from build123d import *

# Parameters (mm, degrees)
SKETCH1_W           = 31.75
SKETCH1_H           = 12.7
SKETCH1_W_2         = 30
SKETCH1_H_2         = 7
BOSS_EXTRUDE1_DEPTH = 13
SKETCH4_R           = 1.778
CUT_EXTRUDE3_DEPTH  = 14
SKETCH5_W           = 21
SKETCH5_H           = 41
CUT_EXTRUDE4_DEPTH  = 10
SKETCH6_R           = 7.112
CUT_EXTRUDE5_DEPTH  = 4
SKETCH7_W           = 31.75
SKETCH7_H           = 12.7
CUT_EXTRUDE6_DEPTH  = 6.35
SKETCH8_R           = 1.778
CUT_EXTRUDE7_DEPTH  = 7.65
SKETCH10_R          = 1.905
CUT_EXTRUDE8_DEPTH  = 14
SKETCH11_R          = 3.302
CUT_EXTRUDE9_DEPTH  = 9.525
SKETCH13_W          = 9.525
SKETCH13_H          = 12.7
SKETCH13_R          = 1.778
BOSS_EXTRUDE2_DEPTH = 13
BOSS_EXTRUDE3_DEPTH = 13
SKETCH18_R          = 1.8415
CUT_EXTRUDE10_DEPTH = 14
FILLET1_R           = 9.525
FILLET2_R           = 3.175
FILLET3_R           = 3.175


with BuildPart() as part:
    # Sketch1 → Boss-Extrude1 (new body)
    with BuildSketch(Plane.XY):
        Polygon((31.75, 12.7), (31.75, 0), (31.75, -28.65), (61.75, -28.65), (61.75, 0), (61.75, 12.7), (61.75, 41.35), (31.75, 41.35), align=None)
        with Locations((15.875, 6.35)):
            Rectangle(SKETCH1_W, SKETCH1_H)
        with Locations((46.75, -32.15)):
            Rectangle(SKETCH1_W_2, SKETCH1_H_2)
    extrude(amount=BOSS_EXTRUDE1_DEPTH)

    # Sketch4 → Cut-Extrude3 (cut, through all)
    with BuildSketch(Plane.XY.offset(13)):
        with Locations((41.75, 22.199999832)):
            Circle(SKETCH4_R)
        with Locations((51.75, 22.199999832)):
            Circle(SKETCH4_R)
        with Locations((41.75, -27.800000168)):
            Circle(SKETCH4_R)
        with Locations((51.75, -27.800000168)):
            Circle(SKETCH4_R)
    extrude(amount=-CUT_EXTRUDE3_DEPTH, mode=Mode.SUBTRACT)

    # Sketch5 → Cut-Extrude4 (cut)
    with BuildSketch(Plane.XY.offset(13)):
        with Locations((46.75, -2.800000024)):
            Rectangle(SKETCH5_W, SKETCH5_H)
    extrude(amount=-CUT_EXTRUDE4_DEPTH, mode=Mode.SUBTRACT)

    # Sketch6 → Cut-Extrude5 (cut, through all)
    with BuildSketch(Plane.XY.offset(3)):
        with Locations((46.75, -12.700000168)):
            Circle(SKETCH6_R)
    extrude(amount=-CUT_EXTRUDE5_DEPTH, mode=Mode.SUBTRACT)

    # Sketch7 → Cut-Extrude6 (cut)
    with BuildSketch(Plane(origin=(0, 0, 0), x_dir=(-1, 0, 0), z_dir=(0, 0, -1))):
        with Locations((-15.875, 6.35)):
            Rectangle(SKETCH7_W, SKETCH7_H)
    extrude(amount=-CUT_EXTRUDE6_DEPTH, mode=Mode.SUBTRACT)

    # Sketch8 → Cut-Extrude7 (cut, through all)
    with BuildSketch(Plane(origin=(0, 0, 6.35), x_dir=(-1, 0, 0), z_dir=(0, 0, -1))):
        with Locations((-6.35, 6.35)):
            Circle(SKETCH8_R)
        with Locations((-25.908, 6.35)):
            Circle(SKETCH8_R)
        with Locations((-16.129, 6.35)):
            Circle(SKETCH8_R)
    extrude(amount=-CUT_EXTRUDE7_DEPTH, mode=Mode.SUBTRACT)

    # Sketch10 → Cut-Extrude8 (cut, through all)
    with BuildSketch(Plane(origin=(0, 0, 0), x_dir=(-1, 0, 0), z_dir=(0, 0, -1))):
        with Locations((-46.75, 25.4)):
            Circle(SKETCH10_R)
    extrude(amount=-CUT_EXTRUDE8_DEPTH, mode=Mode.SUBTRACT)

    # Sketch11 → Cut-Extrude9 (cut)
    with BuildSketch(Plane.XY.offset(13)):
        with Locations((46.75, 25.4)):
            Circle(SKETCH11_R)
    extrude(amount=-CUT_EXTRUDE9_DEPTH, mode=Mode.SUBTRACT)

    # Sketch13 → Boss-Extrude2 (add)
    with BuildSketch(Plane.XY.offset(13)):
        with Locations((66.5125, 6.35)):
            Rectangle(SKETCH13_W, SKETCH13_H)
        with Locations((66.5125, 6.35)):
            Circle(SKETCH13_R, mode=Mode.SUBTRACT)
    extrude(amount=-BOSS_EXTRUDE2_DEPTH)

    # Sketch17 → Boss-Extrude3 (add)
    with BuildSketch(Plane.XY.offset(13)):
        with BuildLine():
            ThreePointArc((36.5125, 48.359214074), (28.382403955, 51.726810119), (31.75, 43.596714074))
            Line((31.75, 43.596714074), (31.75, 48.359214074))
            Line((31.75, 48.359214074), (36.5125, 48.359214074))
        make_face()
        with BuildLine():
            Line((31.75, 48.359214074), (31.75, 43.596714074))
            ThreePointArc((31.75, 43.596714074), (35.117596045, 44.991618029), (36.5125, 48.359214074))
            Line((36.5125, 48.359214074), (31.75, 48.359214074))
        make_face()
        with BuildLine():
            Line((31.75, 43.596714074), (31.75, 41.35))
            Line((31.75, 41.35), (41.275, 41.35))
            Line((41.275, 41.35), (41.275, 48.359214074))
            Line((41.275, 48.359214074), (36.5125, 48.359214074))
            ThreePointArc((36.5125, 48.359214074), (35.117596045, 44.991618029), (31.75, 43.596714074))
        make_face()
        with BuildLine():
            Line((31.75, -35.65), (36.5125, -35.65))
            ThreePointArc((36.5125, -35.65), (35.117596045, -32.282403955), (31.75, -30.8875))
            Line((31.75, -30.8875), (31.75, -35.65))
        make_face()
        with BuildLine():
            ThreePointArc((31.75, -30.8875), (28.382403955, -39.017596045), (36.5125, -35.65))
            Line((36.5125, -35.65), (31.75, -35.65))
            Line((31.75, -35.65), (31.75, -30.8875))
        make_face()
    extrude(amount=-BOSS_EXTRUDE3_DEPTH)

    # Sketch18 → Cut-Extrude10 (cut, through all)
    with BuildSketch(Plane.XY.offset(13)):
        with Locations((31.75, -35.65)):
            Circle(SKETCH18_R)
        with Locations((31.75, 48.359214074)):
            Circle(SKETCH18_R)
    extrude(amount=-CUT_EXTRUDE10_DEPTH, mode=Mode.SUBTRACT)

    # Fillet1
    fillet1_edges = [part.edges().sort_by_distance(p)[0] for p in [
        (31.75, 0, 9.675),
        (31.75, 12.7, 9.675),
        (61.75, 41.35, 6.5),
        (61.75, -35.65, 6.5),
    ]]
    fillet(fillet1_edges, radius=FILLET1_R)

    # Fillet2
    fillet2_edges = [part.edges().sort_by_distance(p)[0] for p in [
        (71.275, 0, 6.5),
        (71.275, 12.7, 6.5),
        (61.75, 12.7, 6.5),
        (61.75, 0, 6.5),
        (31.75, -30.8875, 6.5),
        (36.5125, -35.65, 6.5),
        (31.75, 43.596714074, 6.5),
        (41.275, 41.35, 6.5),
        (36.5125, 48.359214074, 6.5),
    ]]
    fillet(fillet2_edges, radius=FILLET2_R)

    # Fillet3
    fillet3_edges = [part.edges().sort_by_distance(p)[0] for p in [
        (41.275, 48.359214074, 6.5),
        (0, 12.7, 9.675),
        (0, 0, 9.675),
    ]]
    fillet(fillet3_edges, radius=FILLET3_R)


solid = part.part
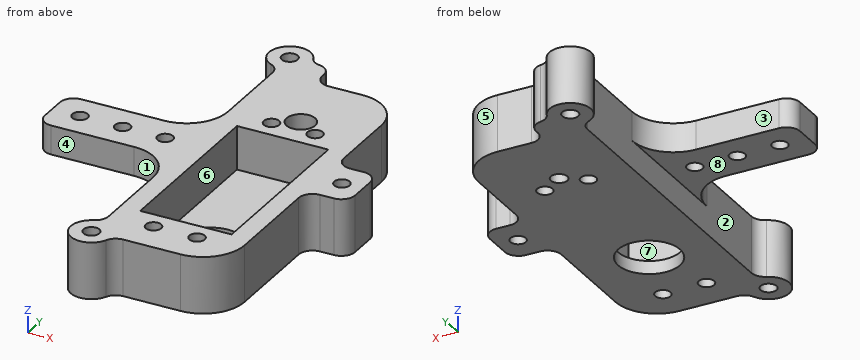
Could you check a few things on this model? Use its own coordinates, in mm. Face numbers are marked on the shaded views. A direction names the side the tool comes from. Give positions to 0.01 mm unless a question says otherwise; leave off trailing zeros. Order: outer loops, then holes, each group sorted by start corner. A loop starts at its lowest first (then second) coordinate and runs counter-clockwise, first axis right, second up. Notation, with made-up numbers: (16.5, -20.5) - (69.5, -20.5) arc R31 cw to (69.5, 7.5) - close; hole circle Ø2 at (15, 83.5). An arc over 180 degrees is marked (long way). One line per item, written item: value. Start each with the question number.
1. Imagine slicing it at C-C on x = 6.35. List the corners of the cut face in (y, z) for me, plus the area to 3 significant figures.
2. For the marked faces 1, 2, 3 and 4, which set-ups out of +Z, -Z, +X, -X, +Y, -Y let a thin tool reach every point of the face, with its end or its side?
3. Imagine slicing it at D-D on y = -12.7. List the corners of the cut face in (x, z) for me, plus the area to 3 significant figures.
4. Imagine slicing it at A-A on x = 46.75. List the corners of the cut face in (y, z) for me (3 decimals).
5. Thinking about a two-plate mould opening in X: for the marked faces 5, 6, 7 and 8, which applies, +X half, -X half, draft (parallel to the pull), parting line (faces both ways), or undercut?
6. For P1, Ø5, axis at x = 60.5, z = 9.5, coming from the -Y side; P2, Ø7.5, axis at x = 14, z = 10.5, coming from the +Y side; P3, Ø1, axis at x = 27, z = 9, coming from the -Y side, each with a flat end and sliding along its axis, tell me the tip position at first contact or that it passes through.
7. Imagine slicing it at B-B on y = 6.35. Give the number of separate pieces and of enclosed holes in the cut face, plus the area to 3 significant figures.
8. If I drill on probe 1 along Y at (x, z) = (27.5, 8.25); probe 2 along Y at (x, z) = (31, 10.5); probe 3 along Y at (x, z) = (28, 6.75), over which ranges is the centre line in solid material (lowest first)?
Values:
1. outline: (0, 6.35) - (4.57, 6.35) - (4.57, 13) - (0, 13) - close; (8.13, 6.35) - (12.7, 6.35) - (12.7, 13) - (8.13, 13) - close
1. area: 60.8 mm²
2. face 1: +Z, -Z, -X
2. face 2: -Z, -X
2. face 3: +Z, -Z, -X, +Y
2. face 4: +Z, -Z, -X, -Y
3. outline: (31.75, 0) - (39.64, 0) - (39.64, 3) - (36.25, 3) - (36.25, 13) - (31.75, 13) - close; (53.86, 0) - (61.75, 0) - (61.75, 13) - (57.25, 13) - (57.25, 3) - (53.86, 3) - close
3. area: 137 mm²
4. outline: (-35.65, 0) - (-19.812, 0) - (-19.812, 3) - (-23.3, 3) - (-23.3, 13) - (-35.65, 13) - close; (-5.588, 0) - (23.495, 0) - (23.495, 3.475) - (22.098, 3.475) - (22.098, 13) - (17.7, 13) - (17.7, 3) - (-5.588, 3) - close; (27.305, 0) - (41.35, 0) - (41.35, 13) - (28.702, 13) - (28.702, 3.475) - (27.305, 3.475) - close
5. face 5: +X half
5. face 6: undercut
5. face 7: undercut
5. face 8: draft
6. P1: y = -33.7
6. P2: y = 12.7
6. P3: y = -37.8
7. separate pieces: 5
7. enclosed holes: 0
7. area: 398 mm²
8. probe 1: -37.8 to -33.5, -1.59 to 5.56, 7.14 to 14.29, 46.21 to 50.51
8. probe 2: -40.35 to -37.33, -33.97 to -30.42, -5.82 to 18.52, 43.13 to 46.68, 50.04 to 53.06
8. probe 3: -38.59 to -32.71, -1.95 to 14.65, 45.42 to 51.3
